from build123d import *

# Parameters (mm, degrees)
SKETCH_W     = 7.75
SKETCH_H     = 7.75
PAD_DEPTH    = 1
SKETCH001_W  = 5.75
SKETCH001_H  = 5.75
PAD001_DEPTH = 4
FILLET_R     = 0.5


with BuildPart() as part:
    # Sketch → Pad (new body)
    with BuildSketch(Plane.XY):
        with Locations((3.875, 3.875)):
            Rectangle(SKETCH_W, SKETCH_H)
    extrude(amount=PAD_DEPTH)

    # Sketch001 (on Face6 of Pad) → Pad001 (join)
    with BuildSketch(Plane.XY.offset(1)):
        with Locations((3.875, 3.875)):
            Rectangle(SKETCH001_W, SKETCH001_H)
    extrude(amount=PAD001_DEPTH)

    # Fillet
    fillet_edges = [part.edges().sort_by_distance(p)[0] for p in [
        (3.875, 6.75, 5),
        (6.75, 3.875, 5),
        (1, 3.875, 5),
        (3.875, 1, 5),
    ]]
    fillet(fillet_edges, radius=FILLET_R)


solid = part.part
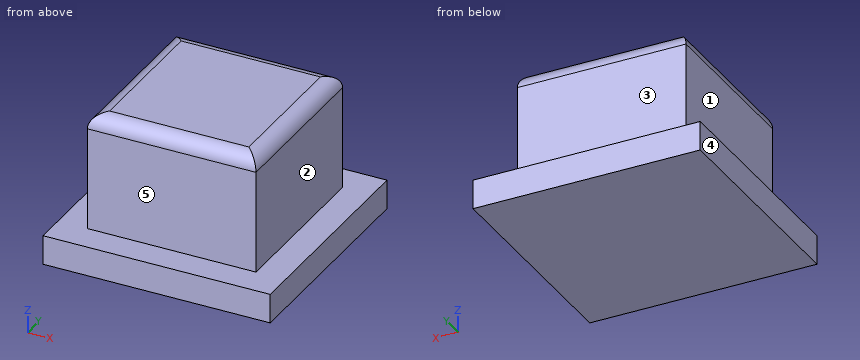
Input: part model. Units: mm. Frame: model coordinates. Face numbers are marked on the shaded views. A direction names the side the tool comes from. Coordinates: 2 decimals unless noted, no trailing zeros. Loops run counter-clockwise (first coordinate to the right, second up) from the corner with the lowest first, then second, coordinate; pieces in that order, holes last. Notation, with made-up numbers: (16.5, 64.5) -> (63.5, 64.5) arc R33 cw to (63.5, 93.5) -> close; hole circle Ø8 at (-23.75, -4.75). An arc over 180 degrees is marked (long way). Write item = value, one per line. Start each with the question number.
Item 1: Cut plane A-A, the plane x = 5.25. Return loops of the section in (y, z), plus the area to 3 significant figures.
Item 2: Material intervals for line 1 (Z direction, x = 7, y = 2.5); line 2 (X direction, y = 4, z = 2.6), sorted ascending.
Item 3: Reachability of the marked faces 1, 2, 3, 4 and 5 from +Z, -Z, +X, -X, +Y, -Y: full face, straight path, thin tool, end or side. Return the list, or none.
Item 4: Cut plane C-C, the plane z = 2.4. Return loops of the section in (x, y).
Item 5: Cut plane D-D, the plane y = 7. Return loops of the section in (x, z), plus the area to 3 significant figures.
Item 6: First-contact query: P1, Ø1, axis at x = 5, z = 3, coming from the +Y side; P2, Ø2, axis at y = 1, z = 4, coming from the -X side; P3, Ø1.8, axis at x = 3, z = 2, coming from the -Y side. Flat tips, straight axial feed; report the tip coordinate or a pass-through.
Ans:
q1.outline = (0, 0) -> (7.75, 0) -> (7.75, 1) -> (6.75, 1) -> (6.75, 4.5) arc R0.5 ccw to (6.25, 5) -> (1.5, 5) arc R0.5 ccw to (1, 4.5) -> (1, 1) -> (0, 1) -> close
q1.area = 30.6 mm²
q2.line_1 = 0 to 1
q2.line_2 = 1 to 6.75
q3.face_1 = +Z, -X, +Y, -Y
q3.face_2 = +Z, +X, +Y, -Y
q3.face_3 = +Z, +X, -X, +Y
q3.face_4 = +Z, -Z, -X, +Y, -Y
q3.face_5 = +Z, +X, -X, -Y
q4.outline = (1, 1) -> (6.75, 1) -> (6.75, 6.75) -> (1, 6.75) -> close
q5.outline = (0, 0) -> (7.75, 0) -> (7.75, 1) -> (0, 1) -> close
q5.area = 7.75 mm²
q6.P1 = 6.75
q6.P2 = 1
q6.P3 = 1
